Could you check a few things on this model? Use its own coordinates, in mm. A direction names the side the tool comes from. Round coordinates to 2 decimals unless told otherwise and drop trailing zeros. Write each loop counter-clockwise with the first axis right and the second up, starting at its lowest first coordinate (ties: lowest second). Pieces come first, ordered by that corner, then holes. Notation, with made-up numbers: M -40,39 L -13,39 A27 ccw -13,69 Z; hole C 32.5,26 d10. An arc over 180 degrees is marked long. One line per item, written item: value. Start each with the question number.
(1) Thinking about a two-plate mould opening in Z: for faces 4 (the face through (-5.724, -1.254, -1.014)), 5 (the face through (-8.41, -1.23, 7.65)), 6 (the face through (3, 3.5, 0)), which applies, released by +Z, released by -Z, zero draft, split by the parting line, or undercut?
(2) I want a section at B-B on y = 0.95. Please give me the cut outline in (x, z).
(3) Which directions (+Z, -Z, +X, -X, +Y, -Y) give clear straight access to the entire face, cutting with the end or side of a thin tool? Please do faces 1 (the face through (-5, -1, 1)), 2 (the face through (-8.6, 1, 0)), 3 (the face through (-7, 2, 4.4)).
(4) I'm going to push flat-ended pins straight in: pin 1 Ø2.5 at (x, z) = (-4, 0) entering from -Y; pin 2 Ø1.5 at (x, y) = (1.5, -1) entering from -Z; pin 3 Ø3.5 at (x, z) = (-4, 4.5) entering from +Y. Where does each tip first touch, or does it pass through?
(5) I want a section at A-A on y = 1.9. Please give me the cut outline in (x, z), and give its area (3 significant figures).
(6) If I drill on L1, parallel to X at y = -0.3, z = 0; L2, parallel to X at y = -0.2, z = 0; L3, parallel to Y at x = -5.5, z = 5.75, over which ranges is the centre line in solid material (lowest first)?
```python
from build123d import *
from OCP.BRepFilletAPI import BRepFilletAPI_MakeChamfer

# Parameters (mm, degrees)
BOSS_EXTRUDE1_DEPTH     = 2
BOSS_EXTRUDE2_START     = 3.5
BOSS_EXTRUDE2_DEPTH     = 3.5
CUT_EXTRUDE1_DEPTH      = 14.883443377
CUT_EXTRUDE1_DEPTH_BACK = 14.883443377
SKETCH4_R               = 1.15
CUT_EXTRUDE2_DEPTH      = 1
CHAMFER1_SIZE           = 0.5
CHAMFER1_SIZE2          = 0.353553391
FILLET1_R               = 3.5
CHAMFER2_SIZE           = 0.5


with BuildPart() as part:
    # Sketch1 → Boss-Extrude1 (new body)
    with BuildSketch(Plane(origin=(0, 0, 0), x_dir=(1, 0, 0), z_dir=(0, 1, 0))):
        with BuildLine():
            Line((-8.6, -4.5), (-8.6, 4.5))
            Line((-8.6, 4.5), (-8.6, 9.5))
            Line((-8.6, 9.5), (0, 9.5))
            ThreePointArc((0, 9.5), (9.5, 0), (0, -9.5))
            Line((0, -9.5), (-8.6, -9.5))
            Line((-8.6, -9.5), (-8.6, -4.5))
        make_face()
    extrude(amount=-BOSS_EXTRUDE1_DEPTH)

    # Sketch2 → Boss-Extrude2 (add)
    with BuildSketch(Plane(origin=(0, 0, 0), x_dir=(1, 0, 0), z_dir=(0, 1, 0)).offset(BOSS_EXTRUDE2_START)):
        Polygon((-8.6, 4.4), (-6.6, 4.4), (-6.6, -4.4), (-8.6, -4.4), (-8.6, 0), align=None)
        with BuildLine():
            Line((-8.4, 9.5), (-5.75, 6.85))
            Line((-5.75, 6.85), (-1.4, 6.85))
            Line((-1.4, 6.85), (-1.4, -6.85))
            Line((-1.4, -6.85), (-5.75, -6.85))
            Line((-5.75, -6.85), (-8.4, -9.5))
            Line((-8.4, -9.5), (0, -9.5))
            ThreePointArc((0, -9.5), (9.5, 0), (0, 9.5))
            Line((0, 9.5), (-8.4, 9.5))
        make_face()
    extrude(amount=-BOSS_EXTRUDE2_DEPTH)

    # Sketch4 → Cut-Extrude1 (cut, two sides: drawn at the far end of the back side and taken through both)
    with BuildSketch(Plane(origin=(0, 0, 0), x_dir=(1, 0, 0), z_dir=(0, 1, 0)).offset(-CUT_EXTRUDE1_DEPTH_BACK)):
        with Locations(Location((-4, 0, 0), (0, 0, 270))):
            Circle(SKETCH4_R)
    extrude(amount=CUT_EXTRUDE1_DEPTH + CUT_EXTRUDE1_DEPTH_BACK, mode=Mode.SUBTRACT)

    # Sketch14 → Cut-Extrude2 (cut)
    with BuildSketch(Plane.XZ.offset(2)):
        Polygon((-5.154700538, 2), (-2.845299462, 2), (-1.690598923, 0), (-2.845299462, -2), (-5.154700538, -2), (-6.309401077, 0), align=None)
    extrude(amount=-CUT_EXTRUDE2_DEPTH, mode=Mode.SUBTRACT)

    # Chamfer1: one chamfer whose edges measure the first distance from different faces: ONE call of the kernel's chamfer builder (chamfer() names one face for all edges)
    chamfer1_edges_1 = [part.edges().sort_by_distance(p)[0] for p in [
        (-8.6, 0, 6.95),
        (-8.6, 1.75, -4.4),
        (-8.6, 1.75, 4.4),
        (-7.6, 3.5, 4.4),
        (-6.6, 3.5, 0),
        (-7.6, 3.5, -4.4),
        (-8.5, 0, -9.5),
        (-1.4, 1.75, -6.85),
        (-1.4, 1.75, 6.85),
        (-7.075, 3.5, -8.175),
        (-3.575, 3.5, -6.85),
        (-1.4, 3.5, 0),
        (-3.575, 3.5, 6.85),
        (-7.075, 3.5, 8.175),
        (-5.732050808, -2, 1),
        (-5.732050808, -2, -1),
        (-4, -2, -2),
        (-2.267949192, -2, -1),
        (-2.267949192, -2, 1),
        (-4, -2, 2),
        (-8.5, 0, 9.5),
        (-8.6, 0, -6.95),
    ]]
    chamfer1_edges_2 = [part.edges().sort_by_distance(p)[0] for p in [
        (-8.4, 1.75, -9.5),
    ]]
    chamfer1_side_2 = [part.faces().sort_by_distance(p)[0] for p in [
        (-7.075, 1.75, -8.175),
    ]]
    chamfer1_edges_3 = [part.edges().sort_by_distance(p)[0] for p in [
        (-8.4, 1.75, 9.5),
    ]]
    chamfer1_side_3 = [part.faces().sort_by_distance(p)[0] for p in [
        (-4.236909871, 0.734978541, 9.5),
    ]]
    chamfer1 = BRepFilletAPI_MakeChamfer(part.part.solid().wrapped)
    for e in chamfer1_edges_1:
        chamfer1.Add(CHAMFER1_SIZE, e.wrapped)
    for e in chamfer1_edges_2:
        chamfer1.Add(CHAMFER1_SIZE, CHAMFER1_SIZE2, e.wrapped, chamfer1_side_2[0].wrapped)  # the first distance lies on this face
    for e in chamfer1_edges_3:
        chamfer1.Add(CHAMFER1_SIZE, CHAMFER1_SIZE2, e.wrapped, chamfer1_side_3[0].wrapped)  # the first distance lies on this face
    add(Compound.cast(chamfer1.Shape()), mode=Mode.REPLACE)

    # Fillet1
    # the kernel refuses this fillet: 3.5 mm, written as the material it takes off along each edge
    with BuildSketch(Plane(origin=(0, -2, 9.5), x_dir=(0, 1, 0), z_dir=(-1, 0, 0))) as fillet1_piece_1:
        with BuildLine():
            CenterArc((FILLET1_R, FILLET1_R), FILLET1_R, 180, 90)
            Line((0, FILLET1_R), (0, 0))
            Line((0, 0), (FILLET1_R, 0))
        make_face()
    extrude(amount=17.35, mode=Mode.SUBTRACT)
    with BuildSketch(Plane(origin=(-17.35, -2, -9.5), x_dir=(0, 0, 1), z_dir=(1, 0, 0))) as fillet1_piece_2:
        with BuildLine():
            CenterArc((FILLET1_R, -FILLET1_R), FILLET1_R, 90, 90)
            Line((0, -FILLET1_R), (0, 0))
            Line((0, 0), (FILLET1_R, 0))
        make_face()
    extrude(amount=17.35, mode=Mode.SUBTRACT)
    with BuildSketch(Plane(origin=(0, -2, 0), x_dir=(0, 0, -1), z_dir=(-1, 0, 0))) as fillet1_piece_3:
        with BuildLine():
            CenterArc((9.5 - FILLET1_R, -FILLET1_R), FILLET1_R, 0, 90)
            Line((9.5, -FILLET1_R), (9.5, 0))
            Line((9.5, 0), (9.5 - FILLET1_R, 0))
        make_face()
    revolve(axis=Axis((0, -2, 0), (0, -1, 0)), revolution_arc=180, mode=Mode.SUBTRACT)

    # Chamfer2
    chamfer2_edges = [part.edges().sort_by_distance(p)[0] for p in [
        (-8.6, -1.602418411, -7.620185175),
        (-8.6, -1.602418411, 7.620185175),
        (-8.6, -2, 0),
    ]]
    chamfer(chamfer2_edges, length=CHAMFER2_SIZE)


solid = part.part
```
Found:
1. face 4: undercut
1. face 5: released by +Z
1. face 6: zero draft
2. outline: M -8.6,-3.9 L -8.1,-4.4 L -6.6,-4.4 L -6.6,4.4 L -8.1,4.4 L -8.6,3.9 Z; M -8.15,9.25 L -5.75,6.85 L -1.9,6.85 L -1.4,6.35 L -1.4,-6.35 L -1.9,-6.85 L -5.75,-6.85 L -8.05,-9.15 L -8.05,-9.46 L 0,-9.46 A9.46 ccw 0,9.46 L -7.94,9.46 Z
3. face 1: -Y
3. face 2: +Z, -Z, -X, +Y, -Y
3. face 3: -X, +Y
4. pin 1: stops at y = -1
4. pin 2: stops at z = -8.92
4. pin 3: stops at y = 0
5. outline: M -8.6,-3.9 L -8.1,-4.4 L -6.6,-4.4 L -6.6,4.4 L -8.1,4.4 L -8.6,3.9 Z; M -8.15,9.25 L -5.75,6.85 L -1.9,6.85 L -1.4,6.35 L -1.4,-6.35 L -1.9,-6.85 L -5.75,-6.85 L -8.05,-9.15 L -8.05,-9.5 L 0,-9.5 A9.5 ccw 0,9.5 L -7.9,9.5 Z
5. area: 216 mm²
6. L1: x = -8.6 to -5.15, -2.85 to 9
6. L2: x = -8.6 to -5.15, -2.85 to 9.06
6. L3: y = -2 to 0
